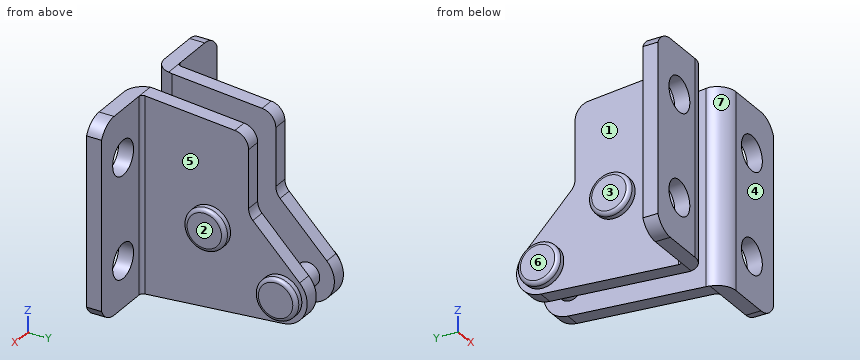
Autodesk Inventor part; units mm, degrees
ref_plane "WF1_XY" through (0, 20.6, 5.007) normal (1, 0, 0) x (0, 0, -1)
ref_plane "WF1_YZ" through (0, 20.6, 5.007) normal (0, 0, -1) x (0, 1, 0)
ref_plane "WF1_ZX" through (0, 20.6, 5.007) normal (0, 1, 0) x (1, 0, 0)
sketch "Skizze_1" plane through (0, 0, 0) normal (0, 0, 1) x (1, 0, 0)
  arc A0 (2, 2.5) -> (4.5, 0) centre (4.5, 2.5) ccw
  line L0 (4.5, 0) -> (12.75, 0)
  line L1 (12.75, 0) -> (12.75, 2)
  line L2 (12.75, 2) -> (4.5, 2)
  arc A1 (4, 2.5) -> (4.5, 2) centre (4.5, 2.5) ccw
  line L3 (4, 2.5) -> (4, 30)
  line L4 (4, 30) -> (2, 30)
  line L5 (2, 30) -> (2, 2.5)
extrude "Extrusion1" add sketch "Skizze_1" along normal blind 26
sketch "Skizze_2" plane through (0, 0, 5.007) normal (0, 0, 1) x (1, 0, 0)
  line L0 (5.17, 20.6) -> (0, 20.6)
  line L1 (-5.17, 20.6) -> (-5.17, 22.89)
  arc A0 (-4.67, 23.39) -> (-5.17, 22.89) centre (-4.67, 22.89) ccw
  line L2 (-4.67, 23.39) -> (-4, 23.39)
  line L3 (-4, 23.39) -> (-4, 22.15)
  line L4 (-4, 22.15) -> (4, 22.15)
  line L5 (4, 22.15) -> (4, 23.39)
  line L6 (4, 23.39) -> (4.67, 23.39)
  arc A1 (5.17, 22.89) -> (4.67, 23.39) centre (4.67, 22.89) ccw
  line L7 (5.17, 22.89) -> (5.17, 20.6)
  line L8 (5.17, 20.6) -> (-5.17, 20.6)
revolve "Revolution1" add sketch "Skizze_2" angle 360 about axis through (5.17, 20.6, 5.007) along (1, 0, 0)
sketch "Skizze_3" plane through (0, 0, 11.357) normal (0, 0, 1) x (1, 0, 0)
  line L0 (5.17, 11.1) -> (0, 11.1)
  line L1 (-5.17, 11.1) -> (-5.17, 13.39)
  arc A0 (-4.67, 13.89) -> (-5.17, 13.39) centre (-4.67, 13.39) ccw
  line L2 (-4.67, 13.89) -> (-4, 13.89)
  line L3 (-4, 13.89) -> (-4, 12.65)
  line L4 (-4, 12.65) -> (4, 12.65)
  line L5 (4, 12.65) -> (4, 13.89)
  line L6 (4, 13.89) -> (4.67, 13.89)
  arc A1 (5.17, 13.39) -> (4.67, 13.89) centre (4.67, 13.39) ccw
  line L7 (5.17, 13.39) -> (5.17, 11.1)
  line L8 (5.17, 11.1) -> (-5.17, 11.1)
revolve "Revolution2" add sketch "Skizze_3" angle 360 about axis through (5.17, 11.1, 11.357) along (1, 0, 0)
sketch "Skizze_5" plane through (0, 0, 0) normal (0, 0, 1) x (1, 0, 0)
  line L0 (-12.75, 2) -> (-12.75, 0)
  line L1 (-12.75, 0) -> (-4.5, 0)
  arc A0 (-4.5, 0) -> (-2, 2.5) centre (-4.5, 2.5) ccw
  line L2 (-2, 2.5) -> (-2, 30)
  line L3 (-2, 30) -> (-4, 30)
  line L4 (-4, 30) -> (-4, 2.5)
  arc A1 (-4.5, 2) -> (-4, 2.5) centre (-4.5, 2.5) ccw
  line L5 (-4.5, 2) -> (-12.75, 2)
extrude "Extrusion2" add sketch "Skizze_5" along normal blind 26
sketch "Skizze_6" plane through (0, 0, 0) normal (1, 0, 0) x (0, 1, 0)
  line L0 (-41, 77) -> (-41, -76)
  line L1 (-41, -76) -> (70, -76)
  line L2 (70, -76) -> (70, 77)
  line L3 (70, 77) -> (-41, 77)
  line L4 (2, 26) -> (0, 26)
  line L5 (0, 26) -> (0, 0)
  line L6 (0, 0) -> (2, 0)
  line L7 (2, 0) -> (20.8805, 1.5183)
  arc A0 (20.8805, 1.5183) -> (23.1011, 7.4554) centre (20.6, 5.007) ccw
  line L8 (23.1011, 7.4554) -> (16.8708, 13.8197)
  arc A1 (16.3, 15.2188) -> (16.8708, 13.8197) centre (18.3, 15.2188) ccw
  line L9 (16.3, 15.2188) -> (16.3, 22.9162)
  arc A2 (16.3, 22.9162) -> (14.4743, 24.9086) centre (14.3, 22.9162) ccw
  line L10 (14.4743, 24.9086) -> (2, 26)
extrude "Extrusion3" cut sketch "Skizze_6" along normal mid plane 100
sketch "Skizze_7" plane through (0, 0, 0) normal (0, 1, 0) x (-1, 0, 0)
  line L0 (50, 50) -> (-61, 50)
  line L1 (-61, 50) -> (-61, -33)
  line L2 (-61, -33) -> (50, -33)
  line L3 (50, -33) -> (50, 50)
  arc A0 (13, 23) -> (10, 26) centre (10, 23) ccw
  line L4 (10, 26) -> (-10, 26)
  arc A1 (-10, 26) -> (-13, 23) centre (-10, 23) ccw
  line L5 (-13, 23) -> (-13, 3)
  arc A2 (-13, 3) -> (-10, 0) centre (-10, 3) ccw
  line L6 (-10, 0) -> (10, 0)
  arc A3 (10, 0) -> (13, 3) centre (10, 3) ccw
  line L7 (13, 3) -> (13, 23)
extrude "Extrusion4" cut sketch "Skizze_7" along normal blind 2
sketch "Skizze_8_ALT_Drilling_1" plane through (0, 0, 0) normal (0, 1, 0) x (-1, 0, 0)
  circle A0 centre (-8, 6.15) radius 2.3
extrude "Extrusion5" cut sketch "Skizze_8_ALT_Drilling_1" along normal blind 2
sketch "Skizze_9_ALT_Drilling_2" plane through (0, 0, 0) normal (0, 1, 0) x (-1, 0, 0)
  circle A0 centre (-8, 19.65) radius 2.3
extrude "Extrusion6" cut sketch "Skizze_9_ALT_Drilling_2" along normal blind 2
sketch "Skizze_10_ALT_Drilling_3" plane through (0, 0, 0) normal (0, 1, 0) x (-1, 0, 0)
  circle A0 centre (8, 6.15) radius 2.3
extrude "Extrusion7" cut sketch "Skizze_10_ALT_Drilling_3" along normal blind 2
sketch "Skizze_11_ALT_Drilling_4" plane through (0, 0, 0) normal (0, 1, 0) x (-1, 0, 0)
  circle A0 centre (8, 19.65) radius 2.3
extrude "Extrusion8" cut sketch "Skizze_11_ALT_Drilling_4" along normal blind 2
ref_plane "WF1_XY" through (0, 20.6, 5.007) normal (1, 0, 0) x (0, 0, -1)
ref_plane "WF1_YZ" through (0, 20.6, 5.007) normal (0, 0, -1) x (0, 1, 0)
ref_plane "WF1_ZX" through (0, 20.6, 5.007) normal (0, 1, 0) x (1, 0, 0)
ref_plane "WF2_XY" through (0, 11.1, 11.357) normal (1, 0, 0) x (0, 0, -1)
ref_plane "WF2_YZ" through (0, 11.1, 11.357) normal (0, 0, -1) x (0, 1, 0)
ref_plane "WF2_ZX" through (0, 11.1, 11.357) normal (0, 1, 0) x (1, 0, 0)
properties part number "305-U-W"
Can you work these out from the model? Positions are in its coordinate system, mm. Face numbers are marked on the shaded views. A direction names the side the tool comes from. Coordinates: 2 decimals unless noted, no trailing zeros. Write each loop counter-clockwise with the first axis right and the second up, starting at its lowest first coordinate (ties: lowest second). Pieces come first, ordered by that corner, then holes. Notation, with made-up numbers: (35, -37) - (78, -37) arc R22 ccw to (78, -14) - close; hole circle Ø1 at (3.5, -37). An arc over 180 degrees is marked (long way). Return JSON: item names as keys, results as strings.
Q1. On a 3-axis mill with a long thin cutter (end or side, diameter ignored), from which of +Z, -Z, +X, -X, +Y, -Y can I reach the whole of each face in a straight line? I mean the marked faces 1, 2, 3 and 4. Say none if no direction works.
Computed values:
{"face 1": "-X", "face 2": "+Z, -Z, +X, +Y", "face 3": "+Z, -Z, -X, +Y", "face 4": "+Z, -Z, +X, -X, -Y"}
Q2. I'm going to push flat-ended pins straight in: pin 1 Ø6.5 at (x, z) = (-9.5, 9.5) entering from +Y; pin 2 Ø6 at (x, y) = (2, 10) entering from +Z; pin 3 Ø2.5 at (y, z) = (12, 11.5) entering from +X; pin 4 Ø12 at (y, z) = (6, 16.5) entering from +X. Where does each tip first touch, or does it pass through?
Computed values:
{"pin 1": "stops at y = 2", "pin 2": "stops at z = 25.56", "pin 3": "stops at x = 5.17", "pin 4": "stops at x = 12.75"}
Q3. If we section it at A-A (x = -8): Please give me the cut outline in (y, z), then the cut area to 3 significant figures.
Computed values:
{"outline": "(0, 0) - (2, 0) - (2, 3.85) - (0, 3.85) - close; (0, 8.45) - (2, 8.45) - (2, 17.35) - (0, 17.35) - close; (0, 21.95) - (2, 21.95) - (2, 26) - (0, 26) - close", "area": "33.6 mm2"}
Q4. Please list where these lines run through material, in increasing order: L1, parallel to Z at x = 8, y = 1.45; L2, parallel to X at y = 13.5, z = 16.25; L3, parallel to Y at x = 7.5, z = 22.25. Write a range as from..to.
Computed values:
{"L1": "z = 0..3.85, 8.45..17.35, 21.95..26", "L2": "x = -4..-2, 2..4", "L3": "y = 0..2"}
Q5. If we section it at D-D (y = 11.1): Please give me the cut outline in (x, z), then the cut area to 3 significant figures.
Computed values:
{"outline": "(-5.17, 9.07) arc R0.5 ccw to (-4.67, 8.57) - (-4, 8.57) - (-4, 0.73) - (-2, 0.73) - (-2, 9.81) - (2, 9.81) - (2, 0.73) - (4, 0.73) - (4, 8.57) - (4.67, 8.57) arc R0.5 ccw to (5.17, 9.07) - (5.17, 13.65) arc R0.5 ccw to (4.67, 14.15) - (4, 14.15) - (4, 25.2) - (2, 25.2) - (2, 12.91) - (-2, 12.91) - (-2, 25.2) - (-4, 25.2) - (-4, 14.15) - (-4.67, 14.15) arc R0.5 ccw to (-5.17, 13.65) - close", "area": "123 mm2"}
Q6. If we section it at C-C (y = 7.25): Please give me the cut outline in (x, z).
Computed values:
{"outline": "(-4, 0.42) - (-2, 0.42) - (-2, 25.54) - (-4, 25.54) - close; (2, 0.42) - (4, 0.42) - (4, 25.54) - (2, 25.54) - close"}
Q7. If we section it at B-B (z = 19.65): Please give me the cut outline in (x, y).
Computed values:
{"outline": "(-12.75, 0) - (-10.3, 0) - (-10.3, 2) - (-12.75, 2) - close; (-5.7, 0) - (-4.5, 0) arc R2.5 ccw to (-2, 2.5) - (-2, 16.3) - (-4, 16.3) - (-4, 2.5) arc R0.5 cw to (-4.5, 2) - (-5.7, 2) - close; (2, 2.5) arc R2.5 ccw to (4.5, 0) - (5.7, 0) - (5.7, 2) - (4.5, 2) arc R0.5 cw to (4, 2.5) - (4, 16.3) - (2, 16.3) - close; (10.3, 0) - (12.75, 0) - (12.75, 2) - (10.3, 2) - close"}
Q8. Thinking about a two-plate mould opening in Y: for the marked faces 5, 6 and 7, which applies, +Y half, -Y half, draft (parallel to the pull), parting line (faces both ways), or undercut?
Computed values:
{"face 5": "undercut", "face 6": "draft", "face 7": "-Y half"}
